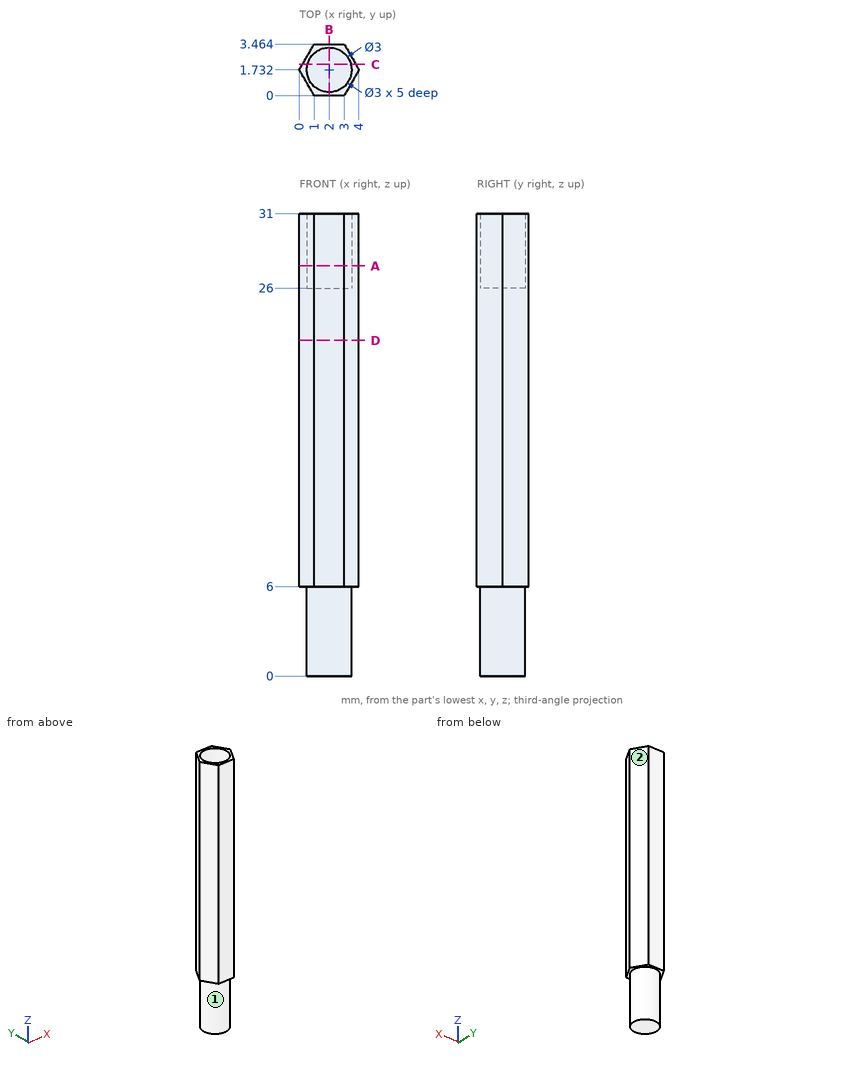
Study the drawing (mm; zero at the part's minimum x, y, z) and answer. A direction names the side the tool comes from. Round coordinates to 2 decimals unless told otherwise and drop trailing zeros. Write each loop counter-clockwise with the first axis right and the second up, starting at its lowest first coordinate (ties: lowest second). Pieces come first, ordered by that corner, then holes. Notation, with made-up numbers: (44, 69) -> (56, 69) arc R26 ccw to (56, 83) -> close; hole circle Ø9 at (56.25, 42.5). An arc over 180 degrees is marked (long way). Write each question's results on one line, items separated by ' | '.
Item 1: Find the intervals of material crossed by line 1 along Y through (x, z) = (2, 28.95); line 2 along Z through (x, y) = (2.05, 1.5); line 3 along Z through (x, y) = (0.95, 3.3), in increasing order. Write a range as [from, to].
Result set:
line 1: [0, 0.23], [3.23, 3.46] | line 2: [0, 26] | line 3: [6, 31]
Item 2: A cutting plane is placed at B-B, the plane x = 2. Determine the outline of the cut face in (y, z), plus the area to 3 significant figures.
Result set:
outline: (0, 6) -> (0.23, 6) -> (0.23, 0) -> (3.23, 0) -> (3.23, 6) -> (3.46, 6) -> (3.46, 31) -> (3.23, 31) -> (3.23, 26) -> (0.23, 26) -> (0.23, 31) -> (0, 31) -> close | area: 89.6 mm^2
Item 3: A cutting plane is placed at D-D, the plane z = 22.5. Determine the outline of the cut face in (x, y), plus the area to 3 significant figures.
Result set:
outline: (0, 1.73) -> (1, 0) -> (3, 0) -> (4, 1.73) -> (3, 3.46) -> (1, 3.46) -> close | area: 10.4 mm^2
Item 4: Which of the six approach directions +Z, -Z, +X, -X, +Y, -Y give full straight-line access (tool end or side, diameter ignored) to the marked faces 1 and 2?
Result set:
face 1: -Z | face 2: +Z, -Z, +X, +Y
Item 5: A cutting plane is placed at C-C, the plane y = 2.1. Determine the outline of the cut face in (x, z).
Result set:
outline: (0.21, 6) -> (0.55, 6) -> (0.55, 0) -> (3.45, 0) -> (3.45, 6) -> (3.79, 6) -> (3.79, 31) -> (3.45, 31) -> (3.45, 26) -> (0.55, 26) -> (0.55, 31) -> (0.21, 31) -> close
Item 6: A cutting plane is placed at A-A, the plane z = 27.5. Determine the outline of the cut face in (x, y).
Result set:
outline: (0, 1.73) -> (1, 0) -> (3, 0) -> (4, 1.73) -> (3, 3.46) -> (1, 3.46) -> close; hole circle Ø3 at (2, 1.73)
Item 7: Flat-ended cylindrical pins translate along their axes: P1, Ø0.9, axis at x = 1.5, y = 1.5, coming from the +Z side; P2, Ø1, axis at y = 2.5, z = 23.5, coming from the +X side (1 decimal). Find the tip coordinate at first contact, or state that the pin passes through.
Result set:
P1: z = 26 | P2: x = 3.8
